```python
from build123d import *

# Parameters (mm, degrees)
F0_W     = 200
F0_H     = 81
F1_DEPTH = 3
F2_W     = 200
F2_H     = 6
F2_H_2   = 5
F3_DEPTH = 1.8
F4_R     = 2
F5_W     = 2.5
F5_H     = 50
F5_W_2   = 60
F5_H_2   = 2.5
F6_DEPTH = 25


with BuildPart() as f1:
    # F0 (on Front) → F1 (new body)
    with BuildSketch(Plane.XZ):
        Rectangle(F0_W, F0_H)
    extrude(amount=F1_DEPTH)

    # F2 (on face) → F3 (cut)
    with BuildSketch(Plane.XZ.offset(3)):
        with Locations((0, 37.5)):
            Rectangle(F2_W, F2_H)
        with Locations((0, -38)):
            Rectangle(F2_W, F2_H_2)
    extrude(amount=-F3_DEPTH, mode=Mode.SUBTRACT)

    # F4
    f4_edges = [f1.edges().sort_by_distance(p)[0] for p in [
        (-100, -0.6, -40.5),
        (-100, -0.6, 40.5),
        (100, -0.6, -40.5),
        (100, -0.6, 40.5),
    ]]
    fillet(f4_edges, radius=F4_R)

    # F5 (on face) → F6 (cut)
    with BuildSketch(Plane.XZ.offset(3)):
        with Locations((-94.75, -0.5)):
            Rectangle(F5_W, F5_H)
        with Locations((94.75, -0.5)):
            Rectangle(F5_W, F5_H)
        with Locations((0, -30.25)):
            Rectangle(F5_W_2, F5_H_2)
    extrude(amount=-F6_DEPTH, mode=Mode.SUBTRACT)


solid = f1.part
```
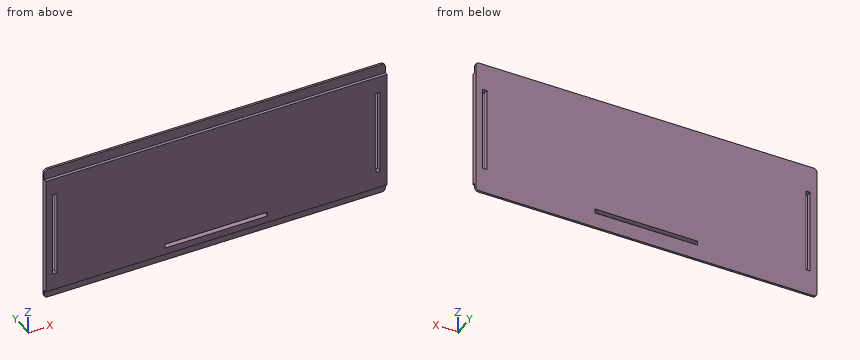
CAD build for the part. Positions are in the model's coordinates, mm. Coordinates: 2 decimals unless noted, no trailing zeros. Loops run counter-clockwise (first coordinate to the right, second up) from the corner with the lowest first, then second, coordinate; pieces in that order, holes last. Notation, with made-up numbers: (57, 5.5) - (97, 5.5) arc R10 ccw to (97, 12.5) - close; hole circle Ø8 at (77.5, 35.25). An arc over 180 degrees is marked (long way). Return JSON: item names as keys, results as strings.
1. Band-saw the part on C-C (y = -1.95). Give the cut face in (x, z).
Result:
{"outline": "(-100, -35.5) - (100, -35.5) - (100, 34.5) - (-100, 34.5) - close; hole (-96, -25.5) - (-93.5, -25.5) - (-93.5, 24.5) - (-96, 24.5) - close; hole (-30, -31.5) - (30, -31.5) - (30, -29) - (-30, -29) - close; hole (93.5, -25.5) - (96, -25.5) - (96, 24.5) - (93.5, 24.5) - close"}
2. Drop flat-ended pins along their axis: pin 1 (0.5 mm diameter, centred on x = 9.5, y = -2, fed in from -Z); pin 2 (1.8 mm diameter, centred on x = -20, z = 38, fed in from -Y); pin 3 (0.9 mm diameter, centred on x = 32.5, y = -2, fed in from +Z). Give the stop position or say it passes through.
Result:
{"pin 1": "stops at z = -35.5", "pin 2": "stops at y = -1.2", "pin 3": "stops at z = 34.5"}
3. Band-saw the part on B-B (x = 4.5). Give the cut face in (y, z).
Result:
{"outline": "(-3, -35.5) - (-1.2, -35.5) - (-1.2, -40.5) - (0, -40.5) - (0, -31.5) - (-3, -31.5) - close; (-3, -29) - (0, -29) - (0, 40.5) - (-1.2, 40.5) - (-1.2, 34.5) - (-3, 34.5) - close"}
4. Band-saw the part on A-A (z = -3.5). Give the cut face in (x, y), and give its area (3 significant figures).
Result:
{"outline": "(-100, -3) - (-96, -3) - (-96, 0) - (-100, 0) - close; (-93.5, -3) - (93.5, -3) - (93.5, 0) - (-93.5, 0) - close; (96, -3) - (100, -3) - (100, 0) - (96, 0) - close", "area": "585 mm2"}
5. Band-saw the part on D-D (x = 74). Give the cut face in (y, z), and give its area (3 significant figures).
Result:
{"outline": "(-3, -35.5) - (-1.2, -35.5) - (-1.2, -40.5) - (0, -40.5) - (0, 40.5) - (-1.2, 40.5) - (-1.2, 34.5) - (-3, 34.5) - close", "area": "223 mm2"}
6. Probe L1, parallel to X at y = -1.1, z = -25; L2, parallel to Z at x = -29, y = -2; L3, parallel to Z at x = 25, y = -0.9. List the from-to ranges inside material, lowest first. Write a range as from..to.
Result:
{"L1": "x = -100..-96, -93.5..93.5, 96..100", "L2": "z = -35.5..-31.5, -29..34.5", "L3": "z = -40.5..-31.5, -29..40.5"}
